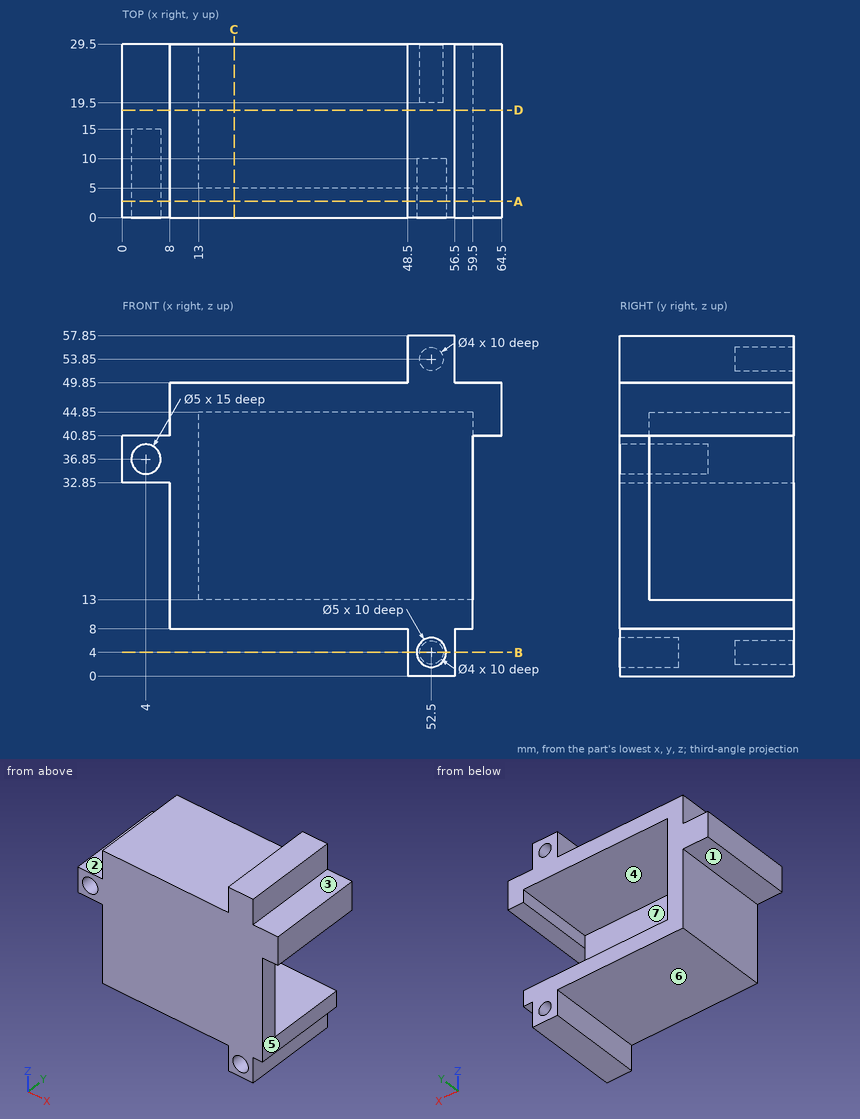
Can you work these out from the drawing? Everything is in mm from the part's minimum corner. A direction names the side the tool comes from. Round coordinates to 2 decimals unless told otherwise and drop trailing zeros. Loops run counter-clockwise (first coordinate to the right, second up) from the corner with the lowest first, then second, coordinate; pieces in that order, holes last. Notation, with made-up numbers: (39, -13) - (48, -13) arc R24 cw to (48, 4) - close; hole circle Ø9 at (48, 5.5). An arc over 180 degrees is marked (long way). Write item = value, one per line. Start each with the question number.
(1) For P1, Ø4, axis at x = 60.5, y = 12.5, coming from the +Z side; P2, Ø4, axis at x = 2, y = 11.5, coming from the +Z side; P3, Ø4, axis at y = 10, z = 27.5, coming from the -X side, each with a flat end and sliding along its axis, tell me the tip position at first contact or that it passes through.
(2) If we mould it in two halves opening along Z, with no side actions, what happens to the marked faces 5, 6 and 7? For each: released by +Z, released by -Z, zero draft, split by the parting line, or undercut.
(3) If we section it at B-B (z = 4): Please give me the cut outline in (x, y), and give its area (3 significant figures).
(4) If we section it at A-A (y = 2.75): Please give me the cut outline in (x, z).
(5) If we section it at C-C (x = 19): Please give me the cut outline in (y, z), and give its area (3 significant figures).
(6) For the marked faces 1, 2, 3 and 4, which set-ups out of +Z, -Z, +X, -X, +Y, -Y let a thin tool reach every point of the face, with its end or its side?
(7) If I drill on probe 1 along X at (y, z) = (20.5, 43); probe 2 along X at (y, z) = (23.25, 4); probe 3 along Z at (x, y) = (27.5, 21.5), over which ranges is the centre line in solid material (lowest first)? Write a range as [from, to].
(8) If we section it at D-D (y = 18.25): Please give me the cut outline in (x, z).
Ans:
q1.P1 = 49.85
q1.P2 = 40.85
q1.P3 = 8
q2.face_5 = zero draft
q2.face_6 = released by -Z
q2.face_7 = undercut
q3.outline = (48.5, 0) - (50, 0) - (50, 10) - (55, 10) - (55, 0) - (56.5, 0) - (56.5, 29.5) - (54.5, 29.5) - (54.5, 19.5) - (50.5, 19.5) - (50.5, 29.5) - (48.5, 29.5) - close
q3.area = 146 mm²
q4.outline = (0, 32.85) - (8, 32.85) - (8, 8) - (48.5, 8) - (48.5, 0) - (56.5, 0) - (56.5, 8) - (59.5, 8) - (59.5, 40.85) - (64.5, 40.85) - (64.5, 49.85) - (56.5, 49.85) - (56.5, 57.85) - (48.5, 57.85) - (48.5, 49.85) - (8, 49.85) - (8, 40.85) - (0, 40.85) - close; hole circle Ø5 at (4, 36.85); hole circle Ø5 at (52.5, 4)
q5.outline = (0, 8) - (29.5, 8) - (29.5, 13) - (5, 13) - (5, 44.85) - (29.5, 44.85) - (29.5, 49.85) - (0, 49.85) - close
q5.area = 454 mm²
q6.face_1 = -Z, -X, +Y, -Y
q6.face_2 = +Z, -X, +Y, -Y
q6.face_3 = +Z, +X, +Y, -Y
q6.face_4 = +Y
q7.probe_1 = [8, 13], [59.5, 64.5]
q7.probe_2 = [48.5, 50.5], [54.5, 56.5]
q7.probe_3 = [8, 13], [44.85, 49.85]
q8.outline = (0, 32.85) - (8, 32.85) - (8, 8) - (48.5, 8) - (48.5, 0) - (56.5, 0) - (56.5, 8) - (59.5, 8) - (59.5, 13) - (13, 13) - (13, 44.85) - (59.5, 44.85) - (59.5, 40.85) - (64.5, 40.85) - (64.5, 49.85) - (56.5, 49.85) - (56.5, 57.85) - (48.5, 57.85) - (48.5, 49.85) - (8, 49.85) - (8, 40.85) - (0, 40.85) - close
